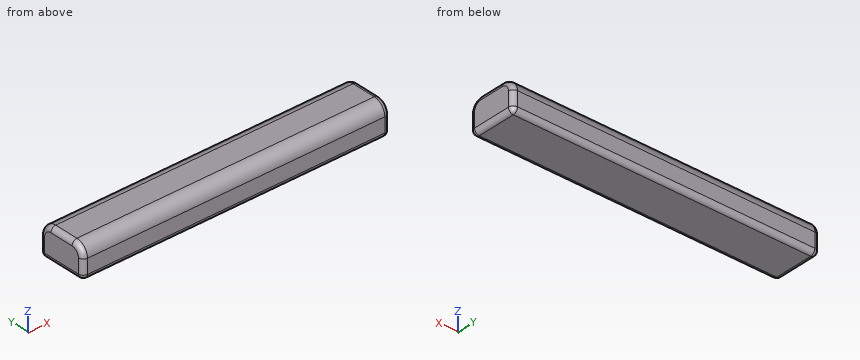
Autodesk Inventor part; units mm, degrees
ref_plane "YZ Plane" through (0, 0, 0) normal (1, 0, 0) x (0, 1, 0)
ref_plane "XZ Plane" through (0, 0, 0) normal (0, 1, 0) x (-1, 0, 0)
ref_plane "XY Plane" through (0, 0, 0) normal (0, 0, 1) x (1, 0, 0)
sketch "Sketch1" plane through (0, 0, 0) normal (0, 0, 1) x (1, 0, 0)
  line L0 (-403.86, 63.5) -> (403.86, 63.5)
  line L1 (403.86, 63.5) -> (403.86, -63.5)
  line L2 (403.86, -63.5) -> (-403.86, -63.5)
  line L3 (-403.86, -63.5) -> (-403.86, 63.5)
  point P0 (0, 0)
  point P1 (-403.86, 0)
  point P2 (0, 63.5)
  dimension "d0" = 807.72
  dimension "d1" = 127
extrude "Extrusion1" add sketch "Sketch1" along normal blind 19.05
sketch "Sketch2" plane through (0, 0, 0) normal (1, 0, 0) x (0, 1, 0)
  line L0 (63.5, 19.05) -> (63.5, 0) construction
  line L1 (63.5, 0) -> (-63.5, 0) construction
  line L2 (-63.5, 0) -> (-63.5, 19.05) construction
  line L3 (-63.5, 19.05) -> (63.5, 19.05) construction
  circle A0 centre (31.75, 50.8) radius 31.75
  circle A1 centre (-31.75, 50.8) radius 31.75
  point P0 (0, 0)
  dimension "d4" = 63.5
  dimension "d5" = 63.5
extrude "Extrusion2" add sketch "Sketch2" along normal mid plane 807.72
sketch "Sketch4" plane through (403.86, -63.5, 0) normal (1, 0, 0) x (0, 0, -1)
  line L0 (-19.05, 127) -> (0, 127)
  line L1 (0, 127) -> (0, 0)
  line L2 (0, 0) -> (-19.05, 0)
  line L3 (-19.05, 0) -> (-19.05, 31.75)
  line L4 (-19.05, 31.75) -> (-19.05, 95.25)
  arc A0 (-50.8, 63.5) -> (-19.05, 95.25) centre (-50.8, 95.25) ccw
  arc A1 (-50.8, 63.5) -> (-19.05, 31.75) centre (-50.8, 31.75) ccw
  arc A2 (-19.05, 31.75) -> (-50.8, 63.5) centre (-50.8, 31.75) ccw
  arc A3 (-19.05, 95.25) -> (-50.8, 63.5) centre (-50.8, 95.25) ccw
  line L5 (-19.05, 95.25) -> (-19.05, 127)
  line L6 (-19.05, 127) -> (-50.8, 127)
  line L7 (-82.55, 95.25) -> (-82.55, 31.75)
  line L8 (-50.8, 0) -> (-19.05, 0)
  point P0 (0, 63.5)
extrude "Extrusion4" add sketch "Sketch4" against normal blind 807.72 contours L5 A3 L6 | L4 A2 A0 | L3 L8 A1 | A1 L7 A3
fillet "Fillet1" radius 12.7 14 edges at (0, 63.5, 0) (403.86, 0, 0) (0, -63.5, 0) (-403.86, 0, 0) (403.86, -63.5, 25.4) (-403.86, -63.5, 25.4) (403.86, -54.2006, 73.2506) (403.86, 0, 82.55) (403.86, 54.2006, 73.2506) (403.86, 63.5, 25.4) (-403.86, -54.2006, 73.2506) (-403.86, 0, 82.55) (-403.86, 54.2006, 73.2506) (-403.86, 63.5, 25.4)
equation "\"d6\" = d0"
equation "\"d10\" = d0"
properties part number "SideBumpers"
CAD build for the part. Positions are in the model's coordinates, mm. Give positions to 0.01 mm unless a question says otherwise; leave off trailing zeros. Order: outer loops, then holes, each group sorted by start corner. A loop starts at its lowest first (then second) coordinate and runs counter-clockwise, first axis right, second up. Notation, with made-up numbers: M 18,55 L 46,55 A18 ccw 46,90 Z; hole C 30,68 d1. An arc over 180 degrees is marked long. Put each result on its own line as item: value. Start each with the question number.
(1) Flat gauge pins, fed straight in: pin 1 Ø8 at (x, z) = (284.5, 65) entering from -Y; pin 2 Ø4 at (x, z) = (-225, 63.5) entering from +Y; pin 3 Ø1 at (y, z) = (22, 73) entering from -X. Where does each tip first touch, or does it go through?
(2) Saw through at A-A, the plane x = -284. Write the cut outline in (y, z).
(3) Drill centre lines: line 1 along Y through (x, z) = (-267.5, 12.5); line 2 along Y through (x, z) = (-45, 53); line 3 along Z through (x, y) = (-151, 53). Where is each one in solid material? Low to high.
Check result:
1. pin 1: stops at y = -61.82
1. pin 2: stops at y = 61.64
1. pin 3: stops at x = -403.58
2. outline: M -63.5,12.7 A12.7 ccw -50.8,0 L 50.8,0 A12.7 ccw 63.5,12.7 L 63.5,50.8 A31.75 ccw 31.75,82.55 L -31.75,82.55 A31.75 ccw -63.5,50.8 Z
3. line 1: y = -63.5 to 63.5
3. line 2: y = -63.42 to 63.42
3. line 3: z = 0.19 to 74.39
